Here's how the part is built. I have some questions about the finished solid (model axes, mm). A direction names the side the tool comes from. Round coordinates to 2 decimals unless told otherwise and drop trailing zeros. Write each loop counter-clockwise with the first axis right and the second up, starting at its lowest first coordinate (ties: lowest second). Pieces come first, ordered by that corner, then holes. Notation, with made-up numbers: (82, 22) -> (113, 22) arc R20 ccw to (113, 45) -> close; hole circle Ø8 at (38.5, 47). An arc over 180 degrees is marked (long way). Put each result on its own line as item: value. Start each with the question number.
1) I want a section at A-A, the plane y = 12.7. List the corners of the cut face in (x, z) for me.
2) I want a section at C-C, the plane z = -5.08. List the corners of the cut face in (x, y) for me.
3) Will these pins go through, and if not, where does the flat tip stop? P1, Ø6, axis at x = 17.5, z = -9, coming from the -Y side; P2, Ø5, axis at y = 14.5, z = -31, coming from the -X side; P3, Ø2, axis at x = 17.5, z = -28, coming from the +Y side.
4) Which directions (+Z, -Z, +X, -X, +Y, -Y) give clear straight access to the entire face, cutting with the end or side of a thin tool? Please do faces 5 (the flat face through (22.86, 10, -4)), 6 (the flat face through (11, 1, -4.064)), 7 (the flat face through (24, 22.86, -5)), 8 (the flat face through (25.4, 1, -19)), 9 (the flat face through (24, 13, -10.16)).
5) We'd pull the mould along Z, two halves only. Please class faces 1 (the flat face through (24, 22.86, -33)), 2 (the flat face through (17, 2, 0)), 3 (the cylindrical face through (24.15, 15.18, -5.63)), 4 (the flat face through (11, 1, -34.036)): released by +Z, released by -Z, zero draft, split by the parting line, or undercut.
6) I want a section at D-D, the plane x = 10.75. List the corners of the cut face in (y, z) for me, then the cut area to 3 significant figures.
7) I want a section at B-B, the plane y = 2. List the corners of the cut face in (x, z) for me.
8) If I drill on line 1 along Z through (x, y) = (24.1, 12.7); line 2 along X through (y, z) = (1.75, -28); line 3 along Y through (x, z) = (23.65, -33.02), over which ranges is the centre line in solid material (lowest first)? Write a range as [from, to].
Autodesk Inventor part; units mm, degrees
ref_plane "YZ Plane" through (0, 0, 0) normal (1, 0, 0) x (0, 1, 0)
ref_plane "XZ Plane" through (0, 0, 0) normal (0, 1, 0) x (-1, 0, 0)
ref_plane "XY Plane" through (0, 0, 0) normal (0, 0, 1) x (1, 0, 0)
sketch "Sketch1" plane through (0, 0, 0) normal (0, 1, 0) x (-1, 0, 0)
  line L0 (0, 0) -> (-25.4, 0)
  line L1 (-25.4, 0) -> (-25.4, -38.1)
  line L2 (-25.4, -38.1) -> (0, -38.1)
  line L3 (0, -38.1) -> (0, 0)
  dimension "d0" = 25.4
  dimension "d1" = 38.1
extrude "Extrusion1" add sketch "Sketch1" along normal blind 2.54
sketch "Sketch3" plane through (0, 2.54, 0) normal (0, 1, 0) x (1, 0, 0)
  line L0 (0, 0) -> (5.08, 0)
  line L1 (5.08, 0) -> (5.08, 4.064)
  line L2 (5.08, 4.064) -> (0, 4.064)
  line L3 (0, 4.064) -> (0, 0)
  line L4 (25.4, 38.1) -> (0, 38.1)
  line L5 (0, 38.1) -> (5.08, 38.1)
  line L6 (5.08, 38.1) -> (5.08, 34.036)
  line L7 (5.08, 34.036) -> (0, 34.036)
  line L8 (0, 34.036) -> (0, 38.1)
  line L9 (5.08, 4.064) -> (16.256, 4.064)
  line L10 (16.256, 4.064) -> (16.256, 34.036)
  line L11 (16.256, 34.036) -> (5.08, 34.036)
  line L12 (5.08, 34.036) -> (5.08, 4.064)
  dimension "d7" = 5.08
  dimension "d8" = 4.064
  dimension "d9" = 5.08
  dimension "d10" = 4.064
  dimension "d11" = 11.176
extrude "Extrusion2" cut sketch "Sketch3" against normal blind 2.54 contours L12 L11 L10 L9
sketch "Sketch4" plane through (0, 2.54, 0) normal (0, 1, 0) x (1, 0, 0)
  line L0 (25.4, 0) -> (25.4, 38.1)
  line L1 (25.4, 0) -> (22.86, 0)
  line L2 (22.86, 0) -> (22.86, 10.16)
  line L3 (22.86, 10.16) -> (25.4, 10.16)
  line L4 (25.4, 10.16) -> (25.4, 0)
  line L5 (25.4, 38.1) -> (22.86, 38.1)
  line L6 (22.86, 38.1) -> (22.86, 27.94)
  line L7 (22.86, 27.94) -> (25.4, 27.94)
  line L8 (25.4, 27.94) -> (25.4, 38.1)
  point P0 (0, 0)
  dimension "d14" = 2.54
  dimension "d15" = 10.16
  dimension "d16" = 2.54
  dimension "d17" = 10.16
extrude "Extrusion3" add sketch "Sketch4" along normal blind 20.32
sketch "Sketch5" plane through (22.86, 2.54, -10.16) normal (-1, 0, 0) x (0, 0, 1)
  line L0 (10.16, 20.32) -> (0, 20.32)
  line L1 (5.08, 20.32) -> (5.08, 10.16)
  point P0 (10.16, -2.54)
  dimension "d20" = 10.16
hole "Hole1" at (22.86, 12.7, -5.08) direction (1, 0, 0) diameter 5.08 end through all
sketch "Sketch6" plane through (22.86, 2.54, -38.1) normal (-1, 0, 0) x (0, 0, 1)
  line L0 (10.16, 20.32) -> (0, 20.32)
  line L1 (5.08, 20.32) -> (5.08, 10.16)
  point P0 (38.1, -2.54)
  dimension "d28" = 10.16
hole "Hole2" at (22.86, 12.7, -33.02) direction (1, 0, 0) diameter 5.08 end through all
properties part number "Actobotics Power Switch Mount v2"
Findings:
1. outline: (22.86, -38.1) -> (25.4, -38.1) -> (25.4, -35.56) -> (22.86, -35.56) -> close; (22.86, -30.48) -> (25.4, -30.48) -> (25.4, -27.94) -> (22.86, -27.94) -> close; (22.86, -10.16) -> (25.4, -10.16) -> (25.4, -7.62) -> (22.86, -7.62) -> close; (22.86, -2.54) -> (25.4, -2.54) -> (25.4, 0) -> (22.86, 0) -> close
2. outline: (0, 0) -> (5.08, 0) -> (5.08, 2.54) -> (0, 2.54) -> close; (16.26, 0) -> (25.4, 0) -> (25.4, 10.16) -> (22.86, 10.16) -> (22.86, 2.54) -> (16.26, 2.54) -> close; (22.86, 15.24) -> (25.4, 15.24) -> (25.4, 22.86) -> (22.86, 22.86) -> close
3. P1: stops at y = 0
3. P2: stops at x = 22.86
3. P3: stops at y = 2.54
4. face 5: +Z, -Z, -X, +Y
4. face 6: +Y, -Y
4. face 7: +Z, -Z, +X, -X, +Y
4. face 8: +Z, -Z, +X, +Y, -Y
4. face 9: +X, -X, +Y
5. face 1: zero draft
5. face 2: released by +Z
5. face 3: undercut
5. face 4: undercut
6. outline: (0, -38.1) -> (2.54, -38.1) -> (2.54, -34.04) -> (0, -34.04) -> close; (0, -4.06) -> (2.54, -4.06) -> (2.54, 0) -> (0, 0) -> close
6. area: 20.6 mm2
7. outline: (0, -38.1) -> (25.4, -38.1) -> (25.4, 0) -> (0, 0) -> close; hole (5.08, -34.04) -> (16.26, -34.04) -> (16.26, -4.06) -> (5.08, -4.06) -> close
8. line 1: z = [-38.1, -35.56], [-30.48, -27.94], [-10.16, -7.62], [-2.54, 0]
8. line 2: x = [0, 5.08], [16.26, 25.4]
8. line 3: y = [0, 10.16], [15.24, 22.86]
